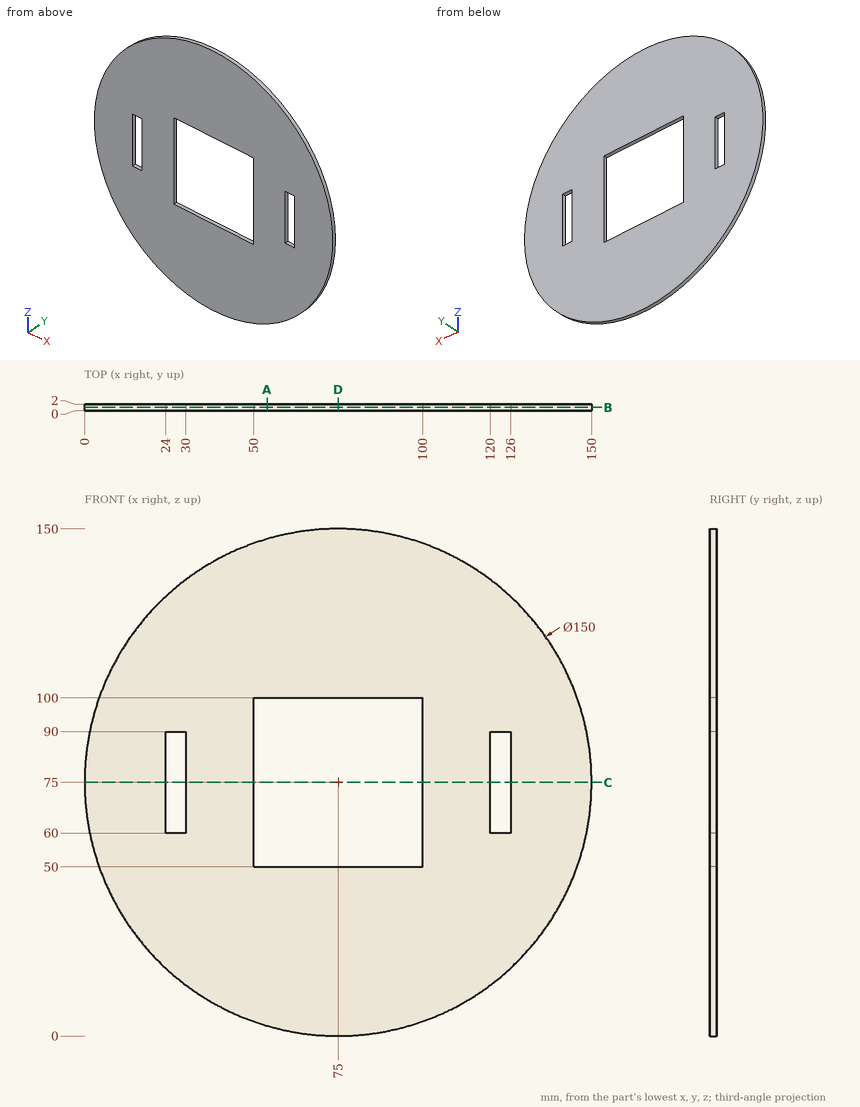
Job drawing, mm, ordinate dimensions from the low corner. One solid piece. Give positions to 0.01 mm unless a question says otherwise; leave off trailing zeros. Loops run counter-clockwise (first coordinate to the right, second up) from the corner with the lowest first, then second, coordinate; pieces in that order, holes last. Notation, with made-up numbers: (75.25, 27.25) -> (95.25, 27.25) arc R17 cw to (95.25, 42.25) -> close; hole circle Ø3 at (69.25, 64). An arc over 180 degrees is marked (long way). Use a Markdown table: item, result. Add a question column.
(1) Slice it at B-B on y = 1. List the corners of the cut face in (x, z), and give its area (3 significant figures).
(2) Slice it at C-C on z = 75. List the corners of the cut face in (x, y).
(3) Slice it at D-D on x = 75. List the corners of the cut face in (y, z), and give its area (3 significant figures).
(4) Wall check: line 1 along X through (y, z) = (1.55, 74); line 2 along X through (y, z) = (1.6, 61); line 3 along Z through (x, y) = (75, 1.4). Give the ranges that are in metal, low to high.
(5) Drop flat-ended pins along their axis: pin 1 Ø1 at (x, y) = (27.5, 1) entering from +Z; pin 2 Ø0.6 at (y, z) = (0.5, 73.5) entering from -X; pin 3 Ø0.6 at (y, z) = (0.5, 68) entering from +X. Give the stop position or say it passes through.
(6) Slice it at A-A on x = 54. List the corners of the cut face in (y, z), and give its area (3 significant figures).
Filled sheet:
| question | item | result |
|---|---|---|
| 1 | outline | circle Ø150 at (75, 75); hole (24, 60) -> (30, 60) -> (30, 90) -> (24, 90) -> close; hole (50, 50) -> (100, 50) -> (100, 100) -> (50, 100) -> close; hole (120, 60) -> (126, 60) -> (126, 90) -> (120, 90) -> close |
| 1 | area | 14,800 mm2 |
| 2 | outline | (0, 0) -> (24, 0) -> (24, 2) -> (0, 2) -> close; (30, 0) -> (50, 0) -> (50, 2) -> (30, 2) -> close; (100, 0) -> (120, 0) -> (120, 2) -> (100, 2) -> close; (126, 0) -> (150, 0) -> (150, 2) -> (126, 2) -> close |
| 3 | outline | (0, 0) -> (2, 0) -> (2, 50) -> (0, 50) -> close; (0, 100) -> (2, 100) -> (2, 150) -> (0, 150) -> close |
| 3 | area | 200 mm2 |
| 4 | line 1 | 0.01 to 24, 30 to 50, 100 to 120, 126 to 149.99 |
| 4 | line 2 | 1.32 to 24, 30 to 50, 100 to 120, 126 to 148.68 |
| 4 | line 3 | 0 to 50, 100 to 150 |
| 5 | pin 1 | z = 133.45 |
| 5 | pin 2 | x = 0.01 |
| 5 | pin 3 | x = 149.7 |
| 6 | outline | (0, 3) -> (2, 3) -> (2, 50) -> (0, 50) -> close; (0, 100) -> (2, 100) -> (2, 147) -> (0, 147) -> close |
| 6 | area | 188 mm2 |
